```python
from build123d import *

# Parameters (mm, degrees)
SKETCH2_R           = 16
BOSS_EXTRUDE1_DEPTH = 4
BOSS_EXTRUDE2_DEPTH = 12
BOSS_EXTRUDE3_DEPTH = 8


with BuildPart() as part:
    # Sketch1 → Revolve1 (revolve)
    with BuildSketch(Plane.XY):
        with BuildLine():
            Line((0, 45), (0, -79))
            ThreePointArc((0, -79), (9.899494937, -74.899494937), (14, -65))
            Line((14, -65), (8, -65))
            Line((8, -65), (8, 45))
            Line((8, 45), (0, 45))
        make_face()
    revolve(axis=Axis((0, 45, 0), (0, -1, 0)))

    # Sketch2 → Boss-Extrude1 (add)
    with BuildSketch(Plane(origin=(0, 45, 0), x_dir=(1, 0, 0), z_dir=(0, 1, 0))):
        Circle(SKETCH2_R)
    extrude(amount=BOSS_EXTRUDE1_DEPTH)

    # Sketch3 → Boss-Extrude2 (add)
    with BuildSketch(Plane(origin=(0, 49, 0), x_dir=(1, 0, 0), z_dir=(0, 1, 0))):
        Polygon((15, 0), (7.5, 12.990381057), (-7.5, 12.990381057), (-15, 0), (-7.5, -12.990381057), (7.5, -12.990381057), align=None)
    extrude(amount=BOSS_EXTRUDE2_DEPTH)

    # Sketch4 → Cut-Revolve1 (revolve, cut)
    with BuildSketch(Plane.XY):
        with BuildLine():
            Line((-11.25, 61), (-11.845920892, 86.206852949))
            Line((-11.845920892, 86.206852949), (-19.210159843, 81.730550841))
            Line((-19.210159843, 81.730550841), (-15, 77.218149523))
            Line((-15, 77.218149523), (-15, 59))
            ThreePointArc((-15, 59), (-14.414213562, 60.414213562), (-13, 61))
            Line((-13, 61), (-11.25, 61))
        make_face()
    revolve(axis=Axis((0, 61, 0), (0, 1, 0)), mode=Mode.SUBTRACT)

    # Sketch5 → Boss-Extrude3 (add)
    with BuildSketch(Plane(origin=(0, 61, 0), x_dir=(1, 0, 0), z_dir=(0, 1, 0))):
        Polygon((14, 0), (7, 12.124355653), (-7, 12.124355653), (-14, 0), (-7, -12.124355653), (7, -12.124355653), align=None)
    extrude(amount=BOSS_EXTRUDE3_DEPTH)

    # Sketch7 → Cut-Revolve4 (revolve, cut)
    with BuildSketch(Plane.XY):
        with BuildLine():
            Line((-10.420461745, 69), (-11.491114181, 93.356215437))
            Line((-11.491114181, 93.356215437), (-17.705025471, 88.394162347))
            Line((-17.705025471, 88.394162347), (-14, 85.377305621))
            Line((-14, 85.377305621), (-14, 67))
            ThreePointArc((-14, 67), (-13.414213562, 68.414213562), (-12, 69))
            Line((-12, 69), (-10.420461745, 69))
        make_face()
    revolve(axis=Axis((0, 69, 0), (0, 1, 0)), mode=Mode.SUBTRACT)


solid = part.part
```
Source: CAD feature listing. Evaluate the final solid. Frame: model axes, mm. A direction names the side the tool comes from. Round coordinates to 2 decimals unless told otherwise and drop trailing zeros. Loops run counter-clockwise (first coordinate to the right, second up) from the corner with the lowest first, then second, coordinate; pieces in that order, holes last. Notation, with made-up numbers: M 12.5,56.5 L 65.5,56.5 A21 cw 65.5,93.5 Z; hole C 20,41 d5. An arc over 180 degrees is marked long. Use a Markdown table: item, result. Add a question column.
1. Ray query, line 1 along X through (y, z) = (19, -6.5); line 2 along Z through (x, y) = (-6, 53); line 3 along Y through (x, z) = (-4, -8.5). Return the intervals inside material, ascending. Write a range as [from, to].
2. Cut plane B-B, the plane y = 7. Output: boundary loops of the cut face in (x, z), and give its area (3 significant figures).
3. Set-up query: faces 5 (the flat face through (10.45, 64.94, 6.15)), 6 (the flat face through (-10.549, 64.942, 5.977)), 7 (the flat face through (-11.198, 54.916, -6.586)), 8 (the flat face through (0, 65, 12.124)). Return all of +Z, -Z, +X, -X, +Y, -Y with unobstructed straight access to the full face (end or side cutting, diameter ignored); none if empty.
4. Contact query for flat-ended pins moving along their axis: pin 1 (8 mm diameter, centred on x = 8.5, y = -44, fed in from +Z); pin 2 (6 mm diameter, centred on x = -4, z = -10.5, fed in from -Y); pin 3 (2 mm diameter, centred on x = -6.5, z = -11, fed in from -Y); pin 4 (5 mm diameter, centred on x = 6, z = 12, fed in from +Y). Output: stop coordinate, or through.
5. Cut plane A-A, the plane y = 56. Output: boundary loops of the cut face in (x, z).
6. Pull-direction query (Y, two-part tool) for faces 1 (the flat face through (6, -65, -6)), 2 (the flat face through (0, 55, 12.99)), 3 (the flat face through (-3.8, 45, -7.3)), 4 (the flat face through (-11, 61, -6)); classes: +Y half, -Y half, draft (parallel to the pull), parting line (faces both ways), or undercut.
Solution:
| question | item | result |
|---|---|---|
| 1 | line 1 | x = [-4.66, 4.66] |
| 1 | line 2 | z = [-12.99, 12.99] |
| 1 | line 3 | y = [-75.38, -65], [45, 69] |
| 2 | outline | C 0,0 d16 |
| 2 | area | 201 mm2 |
| 3 | face 5 | +Z, +X, +Y |
| 3 | face 6 | +Z, -X, +Y |
| 3 | face 7 | -Z, -X, +Y |
| 3 | face 8 | +Z, +X, -X, +Y |
| 4 | pin 1 | stops at z = 6.61 |
| 4 | pin 2 | stops at y = -76.32 |
| 4 | pin 3 | stops at y = -72.57 |
| 4 | pin 4 | stops at y = 69 |
| 5 | outline | M -15,0 L -7.5,-12.99 L 7.5,-12.99 L 15,0 L 7.5,12.99 L -7.5,12.99 Z |
| 6 | face 1 | undercut |
| 6 | face 2 | draft |
| 6 | face 3 | undercut |
| 6 | face 4 | +Y half |
